from build123d import *

# Parameters (mm, degrees)
SKETCH2_R           = 3.35
SKETCH2_R_2         = 1.7
BOSS_EXTRUDE1_DEPTH = 0.3
CIRPATTERN2_COUNT   = 7


with BuildPart() as part:
    # Sketch1 → Revolve1 (revolve)
    with BuildSketch(Plane(origin=(0, 0, 0), x_dir=(0, 0, -1), z_dir=(1, 0, 0))):
        with BuildLine():
            Line((-2.5, 0.625), (-2.5, -0.625))
            ThreePointArc((-2.5, -0.625), (-3.125, 0), (-2.5, 0.625))
        make_face()
    revolve1 = revolve(axis=Axis((0, 0.625, 2.5), (0, -1, 0)))

    # Sketch2 → Boss-Extrude1 (add, symmetric)
    with BuildSketch(Plane(origin=(0, 0, 0), x_dir=(1, 0, 0), z_dir=(0, 1, 0))):
        with Locations(Location((0, 0, 0), (0, 0, 270))):
            Circle(SKETCH2_R)
        with Locations(Location((0, 0, 0), (0, 0, 270))):
            Circle(SKETCH2_R_2, mode=Mode.SUBTRACT)
    extrude(amount=BOSS_EXTRUDE1_DEPTH, both=True)

    # CirPattern2: Revolve1 ×7 about axis
    cirpattern2_axis = Axis((0, 0, 0), (0, 1, 0))
    for i in range(1, CIRPATTERN2_COUNT):
        add(revolve1.rotate(cirpattern2_axis, i * 360 / CIRPATTERN2_COUNT))


solid = part.part
Build history of the part. All positions in model axes, mm. A direction names the side the tool comes from. Coordinates: 2 decimals unless noted, no trailing zeros. Order: outer loops, then holes, each group sorted by start corner. A loop starts at its lowest first (then second) coordinate and runs counter-clockwise, first axis right, second up. Notation, with made-up numbers: (70.25, -33.5) -> (117.25, -33.5) arc R26 cw to (117.25, -19.5) -> close; hole circle Ø10 at (9.25, 45). An arc over 180 degrees is marked (long way). One line per item, written item: value.
(1) Slice it at D-D, the plane y = -0.15. List the corners of the cut face in (x, z), plus the area to 3 significant figures.
Checked values:
outline: circle Ø6.7 at (0, 0); hole circle Ø3.4 at (0, 0)
area: 26.2 mm2
(2) Probe line 1 (X direction, y = -0.1, z = 0); line 2 (Y direction, x = -1.25, z = 1.25); line 3 (Y direction, x = 1.25, z = -2). List the from-to ranges inside material, lowest first. Write a range as [from, to].
Checked values:
line 1: [-3.35, -1.7], [1.7, 3.35]
line 2: [-0.3, 0.3]
line 3: [-0.55, 0.55]
(3) Tool access for faces 1 (the flat face through (-1.4, 0.3, -1.5)), 2 (the flat face through (-1.4, -0.3, -1.5)): list every direction of +Z, -Z, +X, -X, +Y, -Y with a clear straight run to the whole face (end or side of a thin tool).
Checked values:
face 1: +Y
face 2: -Y
(4) Slice it at C-C, the plane y = -0.5. List the corners of the cut face in (x, z) (3 decimals).
Checked values:
outline: circle Ø0.75 at (-2.437, -0.556); circle Ø0.75 at (-1.955, 1.559); circle Ø0.75 at (-1.085, -2.252); circle Ø0.75 at (0, 2.5); circle Ø0.75 at (1.085, -2.252); circle Ø0.75 at (1.955, 1.559); circle Ø0.75 at (2.437, -0.556)
(5) Mould opens along X. For faces 3 (the cylindrical face through (-2.038, 0.004, -2.658)), 4 (the cylindrical face through (-1.66, 0, -0.37)) say: pulls with the +X half, pulls with the -X half, needs draft (parallel to the pull), parting line crosses it, or undercut.
Checked values:
face 3: parting line crosses it
face 4: undercut
(6) Drop a flat-ended pin along its axis: pin 1 Ø1.5 at (x, z) = (0, 1.5) entering from -Y. Give the stop position or say it passes through.
Checked values:
pin 1: y = -0.57
(7) Slice it at B-B, the plane z = 0.25. List the corners of the cut face in (x, y), plus the area to 3 significant figures.
Checked values:
outline: (-3.34, -0.3) -> (-1.68, -0.3) -> (-1.68, 0.3) -> (-3.34, 0.3) -> close; (1.68, -0.3) -> (3.34, -0.3) -> (3.34, 0.3) -> (1.68, 0.3) -> close
area: 1.99 mm2
(8) Slice it at A-A, the plane x = 0. List the corners of the cut face in (y, z) (3 decimals).
Checked values:
outline: (-0.3, -3.35) -> (0.3, -3.35) -> (0.3, -1.7) -> (-0.3, -1.7) -> close; (-0.3, 1.7) -> (0.3, 1.7) -> (0.3, 1.952) arc R0.625 ccw to (0.3, 3.048) -> (0.3, 3.35) -> (-0.3, 3.35) -> (-0.3, 3.048) arc R0.625 ccw to (-0.3, 1.952) -> close
